Build history of the part. All positions in model axes, mm. Give positions to 0.01 mm unless a question says otherwise; leave off trailing zeros. Loops run counter-clockwise (first coordinate to the right, second up) from the corner with the lowest first, then second, coordinate; pieces in that order, holes last.
1) Band-saw the part on B-B on y = 37. List the corners of the cut face in (x, z), then the cut area to 3 significant figures.
2) Band-saw the part on D-D on y = 14. List the corners of the cut face in (x, z), then the cut area to 3 significant figures.
3) Wall check: line 1 (X direction, y = 30, z = 1.2); line 2 (X direction, y = 8.5, z = 2.65); line 3 (X direction, y = -20, z = 0.2). Give the ranges that are in metal, low to high.
4) Flat gauge pins, fed straight in: P1, Ø1.2, axis at x = -38.5, z = 1, coming from the +Y side; P2, Ø1.5, axis at y = -55.5, z = 1, coming from the -X side. Where does each tip first touch, or does it go through?
5) Band-saw the part on C-C on z = 1.55. State how many separate pieces and enclosed holes the cut face has, then the cut area to 3 significant figures.
6) Band-saw the part on A-A on y = -54.5. List the corners of the cut face in (x, z), then the cut area to 3 significant figures.
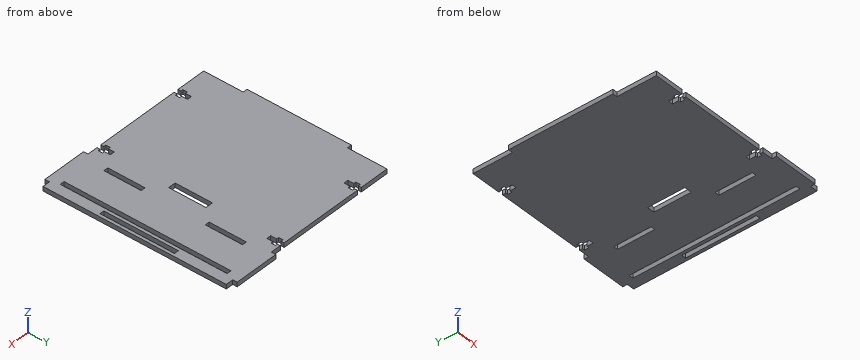
```python
from build123d import *

# Parameters (mm, degrees)
SKETCH1_W           = 5
SKETCH1_H           = 25
SKETCH1_W_2         = 3
SKETCH1_H_2         = 50
SKETCH1_H_3         = 112
BOSS_EXTRUDE2_DEPTH = 3


with BuildPart() as part:
    # Sketch1 → Boss-Extrude2 (new body)
    with BuildSketch(Plane.XY):
        Polygon((17.5, 52.5), (20.5, 52.5), (20.5, 56.5), (22, 56.5), (22, 59.5), (20.5, 59.5), (20.5, 61.5), (27.5, 61.5), (27.5, 64.5), (57.5, 64.5), (57.5, 61.5), (62.5, 61.5), (62.5, -61.5), (57.5, -61.5), (57.5, -64.5), (27.5, -64.5), (27.5, -61.5), (20.5, -61.5), (20.5, -59.5), (22, -59.5), (22, -56.5), (20.5, -56.5), (20.5, -52.5), (17.5, -52.5), (17.5, -56.5), (16, -56.5), (16, -59.5), (17.5, -59.5), (17.5, -61.5), (-39.5, -61.5), (-39.5, -59.5), (-38, -59.5), (-38, -56.5), (-39.5, -56.5), (-39.5, -52.5), (-42.5, -52.5), (-42.5, -56.5), (-44, -56.5), (-44, -59.5), (-42.5, -59.5), (-42.5, -61.5), (-62.5, -61.5), (-62.5, -35), (-65.5, -35), (-65.5, 35), (-62.5, 35), (-62.5, 61.5), (-42.5, 61.5), (-42.5, 59.5), (-44, 59.5), (-44, 56.5), (-42.5, 56.5), (-42.5, 52.5), (-39.5, 52.5), (-39.5, 56.5), (-38, 56.5), (-38, 59.5), (-39.5, 59.5), (-39.5, 61.5), (17.5, 61.5), (17.5, 59.5), (16, 59.5), (16, 56.5), (17.5, 56.5), align=None)
        with Locations((19, 0)):
            Rectangle(SKETCH1_W, SKETCH1_H, mode=Mode.SUBTRACT)
        with Locations((59, 0)):
            Rectangle(SKETCH1_W_2, SKETCH1_H_2, mode=Mode.SUBTRACT)
        with Locations((31, -34)):
            Rectangle(SKETCH1_W_2, SKETCH1_H, mode=Mode.SUBTRACT)
        with Locations((31, 34)):
            Rectangle(SKETCH1_W_2, SKETCH1_H, mode=Mode.SUBTRACT)
        with Locations((54, 0)):
            Rectangle(SKETCH1_W_2, SKETCH1_H_3, mode=Mode.SUBTRACT)
    extrude(amount=BOSS_EXTRUDE2_DEPTH)


solid = part.part
```
Findings below:
1. outline: (-62.5, 0) - (29.5, 0) - (29.5, 3) - (-62.5, 3) - close; (32.5, 0) - (52.5, 0) - (52.5, 3) - (32.5, 3) - close; (55.5, 0) - (62.5, 0) - (62.5, 3) - (55.5, 3) - close
1. area: 357 mm2
2. outline: (-65.5, 0) - (52.5, 0) - (52.5, 3) - (-65.5, 3) - close; (55.5, 0) - (57.5, 0) - (57.5, 3) - (55.5, 3) - close; (60.5, 0) - (62.5, 0) - (62.5, 3) - (60.5, 3) - close
2. area: 366 mm2
3. line 1: x = -65.5 to 29.5, 32.5 to 52.5, 55.5 to 62.5
3. line 2: x = -65.5 to 16.5, 21.5 to 52.5, 55.5 to 57.5, 60.5 to 62.5
3. line 3: x = -65.5 to 52.5, 55.5 to 57.5, 60.5 to 62.5
4. P1: stops at y = 61.5
4. P2: stops at x = -62.5
5. separate pieces: 1
5. enclosed holes: 5
5. area: 14,900 mm2
6. outline: (-62.5, 0) - (-42.5, 0) - (-42.5, 3) - (-62.5, 3) - close; (-39.5, 0) - (17.5, 0) - (17.5, 3) - (-39.5, 3) - close; (20.5, 0) - (52.5, 0) - (52.5, 3) - (20.5, 3) - close; (55.5, 0) - (62.5, 0) - (62.5, 3) - (55.5, 3) - close
6. area: 348 mm2
